The drawing under review shows one solid part. Ordinate dimensions are in mm from its lowest x, y, z. Round coordinates to 2 decimals unless told otherwise and drop trailing zeros. Loops run counter-clockwise (first coordinate to the right, second up) from the corner with the lowest first, then second, coordinate; pieces in that order, holes last. Notation, with made-up numbers: (-6.5, -18) - (38.5, -18) arc R26 ccw to (38.5, -4) - close; hole circle Ø6 at (14, 33.5). An arc over 180 degrees is marked (long way). Answer as CSV lines item,"result".
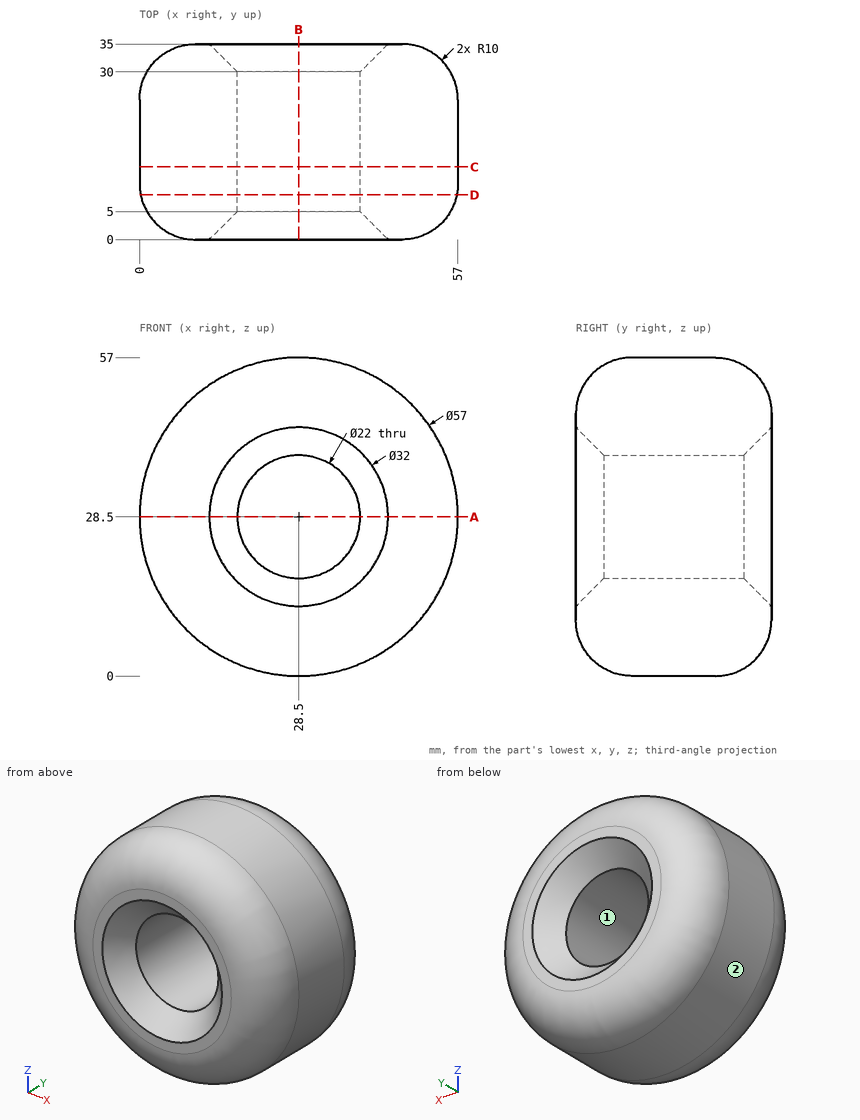
1. Clearance check with flat-ended pins moving along their axes: pin 1 (6 mm diameter, centred on x = 11, z = 47, fed in from +Y); pin 2 (10 mm diameter, centred on y = 8.5, z = 50, fed in from +X); pin 3 (1 mm diameter, centred on x = 46.5, y = 12.5, fed in from -Z); pin 4 (17.5 mm diameter, centred on x = 28.5, z = 28.5, fed in from -Y). State where each tip first meets the part, or that it passes through.
Numbers:
pin 1,"stops at y = 34.18"
pin 2,"stops at x = 51.66"
pin 3,"stops at z = 6.01"
pin 4,"passes through"
2. Take a section at C-C (y = 13). State the section outline as (x, z) points.
Numbers:
outline,"circle Ø57 at (28.5, 28.5); hole circle Ø22 at (28.5, 28.5)"
3. Take a section at D-D (y = 8). State the section outline as (x, z) points, plus the area to 3 significant figures.
Numbers:
outline,"circle Ø56.6 at (28.5, 28.5); hole circle Ø22 at (28.5, 28.5)"
area,"2,140 mm²"
4. Take a section at B-B (x = 28.5). State the section outline as (y, z) points.
Numbers:
outline,"(0, 10) arc R10 ccw to (10, 0) - (25, 0) arc R10 ccw to (35, 10) - (35, 12.5) - (30, 17.5) - (5, 17.5) - (0, 12.5) - close; (0, 44.5) - (5, 39.5) - (30, 39.5) - (35, 44.5) - (35, 47) arc R10 ccw to (25, 57) - (10, 57) arc R10 ccw to (0, 47) - close"
5. Draft analysis for pull direction Z (two halves, no side actions). For the marked faces 1 and 2, state which applies: +Z half, -Z half, draft (parallel to the pull), parting line (faces both ways), or undercut.
Numbers:
face 1,"undercut"
face 2,"parting line"
6. Take a section at A-A (z = 28.5). State the section outline as (x, y) points, plus the area to 3 significant figures.
Numbers:
outline,"(0, 10) arc R10 ccw to (10, 0) - (12.5, 0) - (17.5, 5) - (17.5, 30) - (12.5, 35) - (10, 35) arc R10 ccw to (0, 25) - close; (39.5, 5) - (44.5, 0) - (47, 0) arc R10 ccw to (57, 10) - (57, 25) arc R10 ccw to (47, 35) - (44.5, 35) - (39.5, 30) - close"
area,"1,090 mm²"
7. Wall thickness on probe 1 along Z at (x, y) = (28, 16); probe 2 along Z at (x, y) = (37, 24); probe 3 along X at (y, z) = (30.5, 30): over which ranges is each line inside the solid? List them lowest first.
Numbers:
probe 1,"z = 0 to 17.51, 39.49 to 57"
probe 2,"z = 1.3 to 21.52, 35.48 to 55.7"
probe 3,"x = 1.69 to 17.1, 39.9 to 55.31"
